```python
from build123d import *

# Parameters (mm, degrees)
SKETCH_1_W          = 35
SKETCH_1_H          = 14.4
SKETCH_1_W_2        = 15
SKETCH_1_H_2        = 8.4
EXTRUDE_1_DEPTH     = 3
SKETCH_2_W          = 20
SKETCH_2_H          = 3
CUT_EXTRUDE_1_DEPTH = 1.5
SKETCH_3_R          = 1.45
CUT_EXTRUDE_2_DEPTH = 20
SKETCH_5_R          = 4
CUT_EXTRUDE_4_DEPTH = 10
SKETCH_9_W          = 1.5
SKETCH_9_H          = 14.4
CUT_EXTRUDE_7_DEPTH = 20.159592898
FILLET_2_R          = 2
SKETCH_6_R          = 0.9
CUT_EXTRUDE_5_DEPTH = 1.5
SKETCH_7_R          = 1.45
CUT_EXTRUDE_6_DEPTH = 20.159592898


with BuildPart() as part:
    # 草图1 → 凸台-拉伸1 (new body)
    with BuildSketch(Plane.XY):
        Rectangle(SKETCH_1_W, SKETCH_1_H)
        Rectangle(SKETCH_1_W_2, SKETCH_1_H_2, mode=Mode.SUBTRACT)
    extrude(amount=EXTRUDE_1_DEPTH)

    # 草图2 → 切除-拉伸1 (cut)
    with BuildSketch(Plane.XY.offset(3)):
        Rectangle(SKETCH_2_W, SKETCH_2_H)
    extrude(amount=-CUT_EXTRUDE_1_DEPTH, mode=Mode.SUBTRACT)

    # 草图3 → 切除-拉伸2 (cut)
    with BuildSketch(Plane.XY.offset(3)):
        with Locations((-13, 0)):
            Circle(SKETCH_3_R)
    extrude(amount=-CUT_EXTRUDE_2_DEPTH, mode=Mode.SUBTRACT)

    # 草图5 → 切除-拉伸4 (cut)
    with BuildSketch(Plane.XY.offset(3)):
        with Locations((-14.5, 7.2)):
            Circle(SKETCH_5_R)
        with Locations((14.5, 7.2)):
            Circle(SKETCH_5_R)
        with Locations((-14.5, -7.2)):
            Circle(SKETCH_5_R)
    extrude(amount=-CUT_EXTRUDE_4_DEPTH, mode=Mode.SUBTRACT)

    # 草图9 → 切除-拉伸7 (cut, through all)
    with BuildSketch(Plane.XY.offset(3)):
        with Locations((16.75, 0)):
            Rectangle(SKETCH_9_W, SKETCH_9_H)
    extrude(amount=-CUT_EXTRUDE_7_DEPTH, mode=Mode.SUBTRACT)

    # 圆角2
    fillet_2_edges = [part.edges().sort_by_distance(p)[0] for p in [
        (16, -7.2, 1.5),
        (-10.5, -7.2, 1.5),
        (-17.5, 4.554248689, 1.5),
        (10.5, 7.2, 1.5),
        (-17.5, -4.554248689, 1.5),
        (-10.5, 7.2, 1.5),
        (16, 3.491900756, 1.5),
    ]]
    fillet(fillet_2_edges, radius=FILLET_2_R)

    # 草图6 → 切除-拉伸5 (cut)
    with BuildSketch(Plane.XY.offset(3)):
        with Locations((-9.1, 1.5)):
            Circle(SKETCH_6_R)
        with Locations((-9.1, -1.5)):
            Circle(SKETCH_6_R)
        with Locations((9.1, 1.5)):
            Circle(SKETCH_6_R)
        with Locations((9.1, -1.5)):
            Circle(SKETCH_6_R)
    extrude(amount=-CUT_EXTRUDE_5_DEPTH, mode=Mode.SUBTRACT)

    # 草图7 → 切除-拉伸6 (cut, through all)
    with BuildSketch(Plane.XY.offset(3)):
        with Locations((13, -5)):
            Circle(SKETCH_7_R)
    extrude(amount=-CUT_EXTRUDE_6_DEPTH, mode=Mode.SUBTRACT)


solid = part.part
```
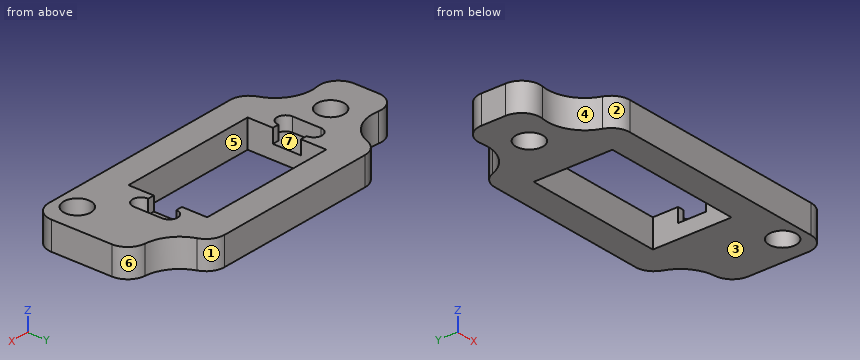
The model under review builds one solid part; all positions refer to its coordinate system, in mm. Face numbers are marked on the shaded views. A direction names the side the tool comes from. Coordinates: 2 decimals unless noted, no trailing zeros. Write each loop counter-clockwise with the first axis right and the second up, starting at its lowest first coordinate (ties: lowest second). Pieces come first, ordered by that corner, then holes. Notation, with made-up numbers: (88.5, -32) - (110.5, -32) arc R24 ccw to (110.5, -10) - close; hole circle Ø3 at (52, 67.5). An arc over 180 degrees is marked (long way). Answer in a Markdown table with one row per item. Add a question column.
Q1. Consider section A-A on x = -6.5. Give the boundary of the cut face in (y, z).
Q2. Consider section B-B on y = 0.75. Give the boundary of the cut face in (x, z), then the cut area to 3 significant figures.
Q3. Clearance check with flat-ended pins moving along their axes: pin 1 (1.2 mm diameter, centred on x = -9, y = 0.5, fed in from +Z); pin 2 (1 mm diameter, centred on x = -11, z = 1, fed in from -Y). State where each tip first meets the part, or that it passes through.
Q4. For the marked faces 5, 6 and 7, list the 3-axis set-ups (+Z, -Z, +X, -X, +Y, -Y) from which the entire face can be reached by the end or side of a thin tool; tool diameter is ignored.
Q5. Consider section C-C on z = 0.3. Give the boundary of the cut face in (x, y).
Q6. To check wall thickness, follow line 1 along Y through (x, z) = (5, 0.65); line 2 along Y through (x, z) = (-8, 2.9); line 3 along X through (y, z) = (4.5, 0.6). State the ranges of each line that lie inside material, in increasing order. Write a range as from..to.
Q7. Draft analysis for pull direction X (two halves, no side actions). For the marked faces 1, 2, 3 and 4, state which applies: +X half, -X half, draft (parallel to the pull), parting line (faces both ways), or undercut.
Q8. Consider section D-D on x = -13. Give the boundary of the cut face in (y, z), then the cut area to 3 significant figures.
Answers below:
| question | item | result |
|---|---|---|
| 1 | outline | (-7.2, 0) - (-4.2, 0) - (-4.2, 3) - (-7.2, 3) - close; (4.2, 0) - (7.2, 0) - (7.2, 3) - (4.2, 3) - close |
| 2 | outline | (-17.5, 0) - (-14.24, 0) - (-14.24, 3) - (-17.5, 3) - close; (-11.76, 0) - (-7.5, 0) - (-7.5, 1.5) - (-10, 1.5) - (-10, 3) - (-11.76, 3) - close; (7.5, 0) - (16, 0) - (16, 3) - (10, 3) - (10, 1.5) - (7.5, 1.5) - close |
| 2 | area | 40.6 mm² |
| 3 | pin 1 | z = 1.5 |
| 3 | pin 2 | y = -6.32 |
| 4 | face 5 | +Z, -Z |
| 4 | face 6 | +Z, -Z, +X, +Y |
| 4 | face 7 | +Z |
| 5 | outline | (-17.5, -1.28) arc R2 ccw to (-15.17, -3.26) arc R4 cw to (-10.73, -5.87) arc R2 ccw to (-8.84, -7.2) - (14, -7.2) arc R2 ccw to (16, -5.2) - (16, 1.22) arc R2 ccw to (14.17, 3.21) arc R4 cw to (10.73, 5.87) arc R2 ccw to (8.84, 7.2) - (-8.84, 7.2) arc R2 ccw to (-10.73, 5.87) arc R4 cw to (-15.17, 3.26) arc R2 ccw to (-17.5, 1.28) - close; hole circle Ø2.9 at (-13, 0); hole (-7.5, -4.2) - (7.5, -4.2) - (7.5, 4.2) - (-7.5, 4.2) - close; hole circle Ø2.9 at (13, -5) |
| 6 | line 1 | -7.2..-4.2, 4.2..7.2 |
| 6 | line 2 | -7.2..-1.5, 1.5..7.2 |
| 6 | line 3 | -11.55..11.55 |
| 7 | face 1 | +X half |
| 7 | face 2 | -X half |
| 7 | face 3 | draft |
| 7 | face 4 | undercut |
| 8 | outline | (-3.49, 0) - (-1.45, 0) - (-1.45, 3) - (-3.49, 3) - close; (1.45, 0) - (3.49, 0) - (3.49, 3) - (1.45, 3) - close |
| 8 | area | 12.3 mm² |
